The listing builds one solid part. Answer for the finished solid, in the listing's coordinates (mm). Face numbers are marked on the shaded views. A direction names the side the tool comes from. Give positions to 0.01 mm unless a question says otherwise; leave off trailing zeros. Order: outer loops, then holes, each group sorted by start corner. A loop starts at its lowest first (then second) coordinate and runs counter-clockwise, first axis right, second up. Notation, with made-up numbers: (21.25, -2) - (44.25, -2) arc R23 cw to (44.25, 24) - close; hole circle Ø8 at (41, 1). An arc over 180 degrees is marked (long way). Answer as a JSON object with one key per item and string values. Group by question number.
Q1. The mould has two halves that part along Y. Classify the marked faces 3, 4 and 5: released by +Y, released by -Y, zero draft, split by the parting line, or undercut.
Q2. A cutting plane is placed at C-C, the plane z = 8.5. Give the vertices of the cut face in (x, y).
Q3. Consider line 1 (Y direction, x = -12, z = 6.5); line 2 (X direction, y = -5, z = 4.5); line 3 (Y direction, x = 12, z = 9). Determine where each line is inside the solid, lowest interval first.
Q4. A cutting plane is placed at B-B, the plane x = -29. Give the vertices of the cut face in (y, z), and give its area (3 significant figures).
Q5. Given pin 1 (10 mm diameter, centred on x = -6.5, y = 2.5, fed in from +Z), flat-ended and moving along its own axis, determine where the tip first touches the part or whether it passes through.
Q6. For the marked faces 1 and 2, determine the directions among +Z, -Z, +X, -X, +Y, -Y from which every point of the face is accessible in a straight line to the end or side of a thin tool.
Q7. A cutting plane is placed at A-A, the plane z = 2.5. Give the vertices of the cut face in (x, y), and give its area (3 significant figures).
Q8. A cutting plane is placed at D-D, the plane y = -11. Give the vertices of the cut face in (x, z).
from build123d import *

# Parameters (mm, degrees)
SKETCH1_W           = 70
SKETCH1_H           = 35
BOSS_EXTRUDE1_DEPTH = 2
SKETCH1_3_W         = 70
SKETCH1_3_H         = 35
SKETCH1_3_W_2       = 66
SKETCH1_3_H_2       = 31
BOSS_EXTRUDE2_DEPTH = 9.5
SKETCH1_4_W         = 55
SKETCH1_4_H         = 20
BOSS_EXTRUDE3_DEPTH = 7.5


with BuildPart() as part:
    # Sketch1 → Boss-Extrude1 (new body)
    with BuildSketch(Plane.XY):
        Rectangle(SKETCH1_W, SKETCH1_H)
    extrude(amount=-BOSS_EXTRUDE1_DEPTH)

    # Sketch1<3> → Boss-Extrude2 (add)
    with BuildSketch(Plane.XY):
        Rectangle(SKETCH1_3_W, SKETCH1_3_H)
        Rectangle(SKETCH1_3_W_2, SKETCH1_3_H_2, mode=Mode.SUBTRACT)
    extrude(amount=BOSS_EXTRUDE2_DEPTH)

    # Sketch1<4> → Boss-Extrude3 (add)
    with BuildSketch(Plane.XY):
        Rectangle(SKETCH1_4_W, SKETCH1_4_H)
    extrude(amount=BOSS_EXTRUDE3_DEPTH)


solid = part.part
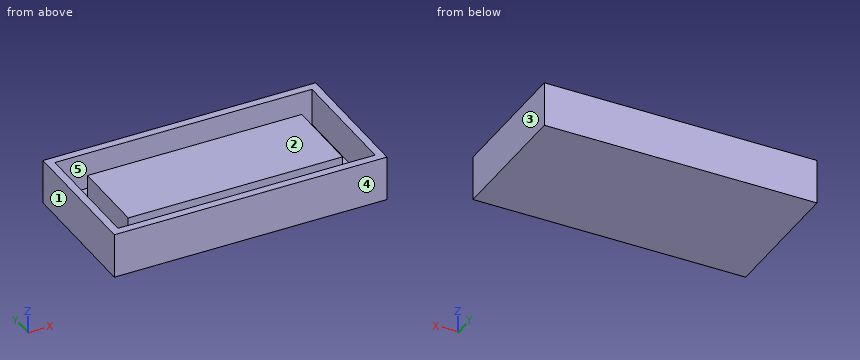
Reply:
{
 "1": {"face 3": "zero draft", "face 4": "released by -Y", "face 5": "undercut"},
 "2": {"outline": "(-35, -17.5) - (35, -17.5) - (35, 17.5) - (-35, 17.5) - close; hole (-33, -15.5) - (33, -15.5) - (33, 15.5) - (-33, 15.5) - close"},
 "3": {"line 1": "y = -17.5 to -15.5, -10 to 10, 15.5 to 17.5", "line 2": "x = -35 to -33, -27.5 to 27.5, 33 to 35", "line 3": "y = -17.5 to -15.5, 15.5 to 17.5"},
 "4": {"outline": "(-17.5, -2) - (17.5, -2) - (17.5, 9.5) - (15.5, 9.5) - (15.5, 0) - (-15.5, 0) - (-15.5, 9.5) - (-17.5, 9.5) - close", "area": "108 mm^2"},
 "5": {"pin 1": "stops at z = 7.5"},
 "6": {"face 1": "+Z, -Z, -X, +Y, -Y", "face 2": "+Z"},
 "7": {"outline": "(-35, -17.5) - (35, -17.5) - (35, 17.5) - (-35, 17.5) - close; (-27.5, -10) - (27.5, -10) - (27.5, 10) - (-27.5, 10) - close; hole (-33, -15.5) - (33, -15.5) - (33, 15.5) - (-33, 15.5) - close", "area": "1,500 mm^2"},
 "8": {"outline": "(-35, -2) - (35, -2) - (35, 9.5) - (33, 9.5) - (33, 0) - (-33, 0) - (-33, 9.5) - (-35, 9.5) - close"}
}
